Work out the finished part from the listing and answer in its coordinate system (mm). A direction names the side the tool comes from. Give positions to 0.01 mm unless a question says otherwise; leave off trailing zeros. Order: outer loops, then holes, each group sorted by start corner. A loop starts at its lowest first (then second) coordinate and runs counter-clockwise, first axis right, second up. Notation, with made-up numbers: (75.5, 72) - (106.5, 72) arc R21 ccw to (106.5, 96) - close; hole circle Ø6 at (45.25, 25). An arc over 180 degrees is marked (long way). Put each result on its own line as item: value.
```python
from build123d import *

# Parameters (mm, degrees)
F1_DEPTH = 10
F3_DEPTH = 10
F4_R     = 115
F5_DEPTH = 6
F6_R     = 5.5
F7_DEPTH = 10


with BuildPart() as f1:
    # F0 (on Front) → F1 (new body)
    with BuildSketch(Plane.XZ):
        with BuildLine():
            Line((-60, 199.5), (-131.5733290036, 122.8350890215))
            ThreePointArc((-131.5733290036, 122.8350890215), (0, -180), (131.5733290036, 122.8350890215))
            Line((131.5733290036, 122.8350890215), (60, 199.5))
            Line((60, 199.5), (0, 199.5))
            Line((0, 199.5), (-60, 199.5))
        make_face()
    extrude(amount=-F1_DEPTH)

    # F2 (on face) → F3 (cut, through all)
    with BuildSketch(Plane.XZ):
        with BuildLine():
            Line((-60, 199.5), (60, 199.5))
            ThreePointArc((60, 199.5), (0, 259.5), (-60, 199.5))
        make_face()
        with BuildLine():
            ThreePointArc((-60, 199.5), (0, 139.5), (60, 199.5))
            Line((60, 199.5), (-60, 199.5))
        make_face()
    extrude(amount=-F3_DEPTH, mode=Mode.SUBTRACT)

    # F4 (on face) → F5 (join)
    with BuildSketch(Plane.XZ):
        Circle(F4_R)
    extrude(amount=F5_DEPTH)

    # F6 (on face) → F7 (cut, through all)
    with BuildSketch(Plane.XZ):
        with Locations((-63.75, 110.4182389825)):
            Circle(F6_R)
        with Locations((0, 127.5)):
            Circle(F6_R)
        with Locations((63.75, 110.4182389825)):
            Circle(F6_R)
        with Locations((110.4182389825, 63.75)):
            Circle(F6_R)
        with Locations((127.5, 0)):
            Circle(F6_R)
        with Locations((110.4182389825, -63.75)):
            Circle(F6_R)
        with Locations((63.75, -110.4182389825)):
            Circle(F6_R)
        with Locations((0, -127.5)):
            Circle(F6_R)
        with Locations((-63.75, -110.4182389825)):
            Circle(F6_R)
        with Locations((-110.4182389825, -63.75)):
            Circle(F6_R)
        with Locations((-127.5, 0)):
            Circle(F6_R)
        with Locations((-110.4182389825, 63.75)):
            Circle(F6_R)
    extrude(amount=-F7_DEPTH, mode=Mode.SUBTRACT)


solid = f1.part
```
(1) Section C-C, the plane x = 85.5 is taken. Write down the section's boundary in (y, z).
Geometry check:
outline: (-6, -76.91) - (0, -76.91) - (0, -158.4) - (10, -158.4) - (10, 172.19) - (0, 172.19) - (0, 76.91) - (-6, 76.91) - close
(2) A tool of negligible diameter and unlimited length cuts with its end or side. For faces 5 (the face through (-43, 0, -114)), 6 (the face through (-1.319, 4.93, 139.515)), from which of +Z, -Z, +X, -X, +Y, -Y can it reach the whole face along a straight path? Write none if from no direction.
Geometry check:
face 5: -Y
face 6: +Z, +Y, -Y
(3) Determine the mould class of faces 1 (the face through (106.365, 4.93, -60.033)), 2 (the face through (96.29, 4.93, 160.63)), 3 (the face through (-5.85, 4.93, -179.905)), 4 (the face through (122, 5, 0)) for opening direction Z: pulls with the +Z half, pulls with the -Z half, needs draft (parallel to the pull), parting line crosses it, or undercut.
Geometry check:
face 1: undercut
face 2: pulls with the +Z half
face 3: parting line crosses it
face 4: undercut
(4) Section A-A, the plane z = 0 is taken. Write down the section's boundary in (x, y).
Geometry check:
outline: (-180, 0) - (-133, 0) - (-133, 10) - (-180, 10) - close; (-122, 0) - (-115, 0) - (-115, -6) - (115, -6) - (115, 0) - (122, 0) - (122, 10) - (-122, 10) - close; (133, 0) - (180, 0) - (180, 10) - (133, 10) - close
(5) Section D-D, the plane y = 6.25 is taken. Count the separate pieces of the cut face and the enclosed holes in it, then the cut area to 3 significant figures.
Geometry check:
separate pieces: 1
enclosed holes: 12
area: 99,300 mm²
(6) Section B-B, the plane z = 127.5 is taken. Write down the section's boundary in (x, y).
Geometry check:
outline: (-127.22, 0) - (-5.5, 0) - (-5.5, 10) - (-127.22, 10) - close; (5.5, 0) - (127.22, 0) - (127.22, 10) - (5.5, 10) - close
(7) Straight lines are drawn through the part: line 1 (Z direction, x = -68, y = 1.25); line 2 (Z direction, x = 63.75, y = 4.75); line 3 (Y direction, x = -86, z = -110). For each, find the intervals that lie inside material, in ascending order.
Geometry check:
line 1: z = -166.66 to -113.91, -106.93 to 106.93, 113.91 to 190.93
line 2: z = -168.33 to -115.92, -104.92 to 104.92, 115.92 to 195.48
line 3: y = 0 to 10
(8) Given pin 1 (4 mm diameter, centred on x = 141.5, z = 33, fed in from -Y); pin 2 (5 mm diameter, centred on y = 7.5, z = -117, fed in from +X); pin 3 (12.5 mm diameter, centred on x = 63.75, z = -110.42, fed in from +Y); pin 4 (6 mm diameter, centred on y = 1.5, z = 109.5, fed in from -X), each flat-ended and moving along its own axis, determine where each tip first touches the part or whether it passes through.
Geometry check:
pin 1: stops at y = 0
pin 2: stops at x = 138.89
pin 3: stops at y = 10
pin 4: stops at x = -145.11
